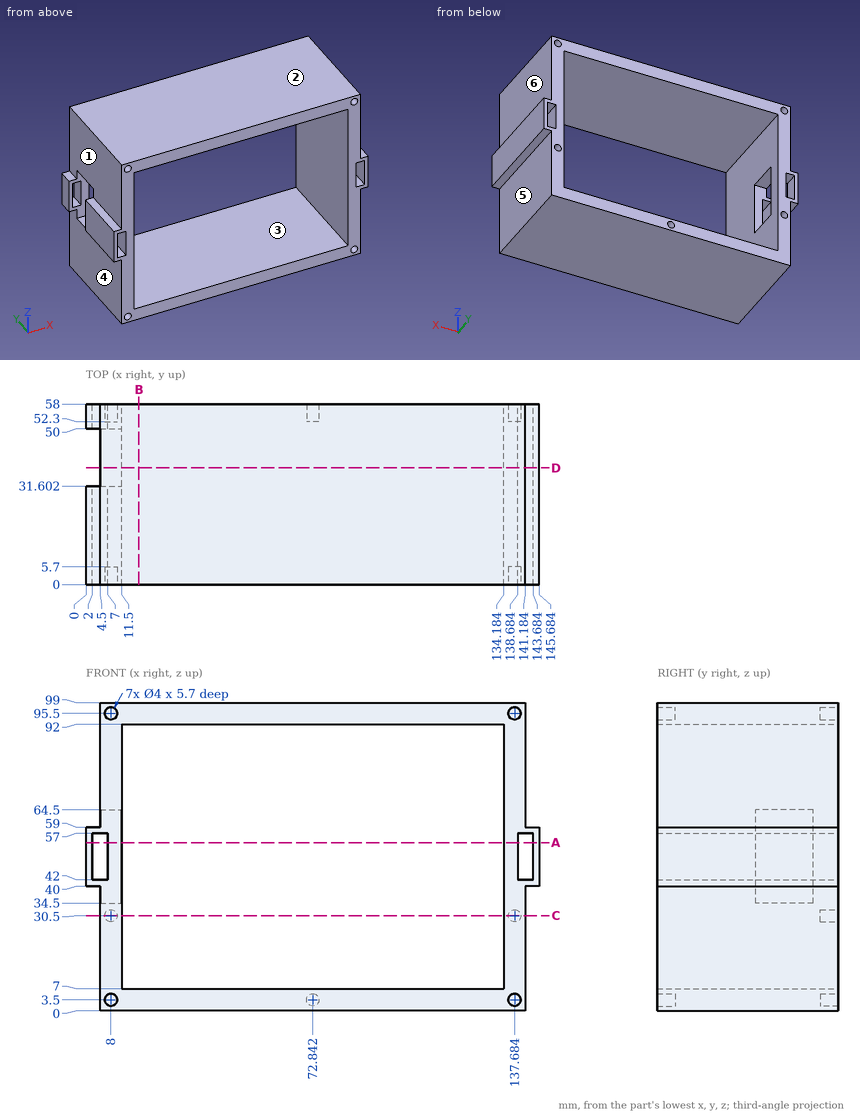
Verification items for this drawing (mm, ordinates from the low corner). A direction names the side the tool comes from. Give positions to 0.01 mm unless a question says otherwise; leave off trailing zeros. Write each loop counter-clockwise with the first axis right and the second up, starting at its lowest first coordinate (ties: lowest second). Pieces come first, ordered by that corner, then holes.
1) Set-up check for the marked faces 4, 5 and 6: record each of +Z, -Z, +X, -X, +Y, -Y from which the full face is reachable in a straight line by a thin tool's end or side.
Values follow:
face 4: -Z, -X, +Y, -Y
face 5: -Z, +X, +Y, -Y
face 6: +Z, +X, +Y, -Y
2) Cross-section at C-C (z = 30.5). Record the boundary of the cut face in (x, y).
Values follow:
outline: (4.5, 0) - (11.5, 0) - (11.5, 58) - (10, 58) - (10, 52.3) - (6, 52.3) - (6, 58) - (4.5, 58) - close; (134.18, 0) - (141.18, 0) - (141.18, 58) - (139.68, 58) - (139.68, 52.3) - (135.68, 52.3) - (135.68, 58) - (134.18, 58) - close
3) Go/stop test with flat-tipped pins: pin 1 Ø1 at (y, z) = (24, 85) entering from -X; pin 2 Ø1.2 at (x, z) = (7.5, 30) entering from +Y; pin 3 Ø5 at (y, z) = (30.5, 82.5) entering from +X. Record where each tip stops, or that it passes through.
Values follow:
pin 1: stops at x = 4.5
pin 2: stops at y = 52.3
pin 3: stops at x = 141.18
4) Cross-section at D-D (y = 37.5). Record the boundary of the cut face in (x, z), plus the area to 3 significant figures.
Values follow:
outline: (4.5, 0) - (141.18, 0) - (141.18, 40) - (145.68, 40) - (145.68, 59) - (141.18, 59) - (141.18, 99) - (4.5, 99) - (4.5, 64.5) - (11.5, 64.5) - (11.5, 92) - (134.18, 92) - (134.18, 7) - (11.5, 7) - (11.5, 34.5) - (4.5, 34.5) - close; hole (138.68, 42) - (143.68, 42) - (143.68, 57) - (138.68, 57) - close
area: 2,900 mm2
5) Cross-section at B-B (x = 17). Record the boundary of the cut face in (y, z).
Values follow:
outline: (0, 0) - (58, 0) - (58, 7) - (0, 7) - close; (0, 92) - (58, 92) - (58, 99) - (0, 99) - close
6) Cross-section at A-A (z = 54). Record the boundary of the cut face in (x, y).
Values follow:
outline: (0, 0) - (2, 0) - (2, 31.6) - (0, 31.6) - close; (0, 50) - (2, 50) - (2, 58) - (0, 58) - close; (7, 0) - (11.5, 0) - (11.5, 31.6) - (7, 31.6) - close; (7, 50) - (11.5, 50) - (11.5, 58) - (7, 58) - close; (134.18, 0) - (138.68, 0) - (138.68, 58) - (134.18, 58) - close; (143.68, 0) - (145.68, 0) - (145.68, 58) - (143.68, 58) - close
7) Release check for a two-part mould opening along X. For the marked faces 1, 2 and 3 record: released by +X, released by -X, zero draft, split by the parting line, or undercut.
Values follow:
face 1: released by -X
face 2: zero draft
face 3: undercut
8) Thickness scan on line 1 (Z direction, x = 8, y = 54.65); line 2 (X direction, y = 53.9, z = 95.5); line 3 (X direction, y = 54.95, z = 3.5). Record the ranges inside material, lowest first.
Values follow:
line 1: z = 0 to 28.5, 32.5 to 93.5, 97.5 to 99
line 2: x = 4.5 to 6, 10 to 135.68, 139.68 to 141.18
line 3: x = 4.5 to 70.84, 74.84 to 141.18
